```python
from build123d import *

# Parameters (mm, degrees)
SKETCH_1_R      = 1.65
EXTRUDE_1_DEPTH = 3


with BuildPart() as part:
    # 草图1 → 凸台-拉伸1 (new body)
    with BuildSketch(Plane.XY):
        Polygon((-55, 10), (-55, -10), (55, -10), (55, 10), (50, 50.05274288), (30, 50.05274288), (25.979309591, 25), (-25.864232627, 25), (-30, 50.05274288), (-50, 50.05274288), align=None)
        with Locations((15, 0)):
            Circle(SKETCH_1_R, mode=Mode.SUBTRACT)
        with Locations((-15, 0)):
            Circle(SKETCH_1_R, mode=Mode.SUBTRACT)
        with Locations((35, 0)):
            Circle(SKETCH_1_R, mode=Mode.SUBTRACT)
        with Locations((-35, 0)):
            Circle(SKETCH_1_R, mode=Mode.SUBTRACT)
        with Locations((45, 0)):
            Circle(SKETCH_1_R, mode=Mode.SUBTRACT)
        with Locations((-45, 0)):
            Circle(SKETCH_1_R, mode=Mode.SUBTRACT)
        with Locations((-40, 20)):
            Circle(SKETCH_1_R, mode=Mode.SUBTRACT)
        with Locations((-40, 30)):
            Circle(SKETCH_1_R, mode=Mode.SUBTRACT)
        with Locations((40, 20)):
            Circle(SKETCH_1_R, mode=Mode.SUBTRACT)
        with Locations((40, 30)):
            Circle(SKETCH_1_R, mode=Mode.SUBTRACT)
        with Locations((-40, 40)):
            Circle(SKETCH_1_R, mode=Mode.SUBTRACT)
        with Locations((40, 40)):
            Circle(SKETCH_1_R, mode=Mode.SUBTRACT)
    extrude(amount=EXTRUDE_1_DEPTH)


solid = part.part
```
Source: CAD feature listing. Evaluate the final solid. Frame: model axes, mm. A direction names the side the tool comes from. Round coordinates to 2 decimals unless told otherwise and drop trailing zeros. Loops run counter-clockwise (first coordinate to the right, second up) from the corner with the lowest first, then second, coordinate; pieces in that order, holes last.
(1) Section query C-C (z = 2.15). Give the number of separate pieces and of enclosed holes in the cut face, and give its area (3 significant figures).
From the geometry:
separate pieces: 1
enclosed holes: 12
area: 4,900 mm2
(2) Section query A-A (x = -35). Output: boundary loops of the cut face in (y, z).
From the geometry:
outline: (-10, 0) - (-1.65, 0) - (-1.65, 3) - (-10, 3) - close; (1.65, 0) - (50.05, 0) - (50.05, 3) - (1.65, 3) - close
(3) Material intervals for probe 1 along Y at (x, z) = (40, 2.3); probe 2 along Y at (x, z) = (-15, 2.15); probe 3 along X at (y, z) = (28.5, 1.05), sorted ascending.
From the geometry:
probe 1: y = -10 to 18.35, 21.65 to 28.35, 31.65 to 38.35, 41.65 to 50.05
probe 2: y = -10 to -1.65, 1.65 to 25
probe 3: x = -52.69 to -40.69, -39.31 to -26.44, 26.54 to 39.31, 40.69 to 52.69
(4) Contact query for a flat-ended pin moving along its axis: pin 1 Ø3 at (x, y) = (-40, 40) entering from -Z. Output: stop coordinate, or through.
From the geometry:
pin 1: passes through
(5) Pull-direction query (X, two-part tool) for faces 1 (the flat face through (52.535, 29.746, 1.479)), 2 (the cylindrical face through (38.35, 20.07, 1.48)), 3 (the flat face through (-52.465, 30.307, 1.479)); classes: +X half, -X half, draft (parallel to the pull), parting line (faces both ways), or undercut.
From the geometry:
face 1: +X half
face 2: undercut
face 3: -X half
(6) Access query for faces 4 (the flat face through (28.018, 37.702, 1.479)), 5 (the cylindrical face through (-36.65, 0.07, 1.48)). Directions: +Z, -Z, +X, -X, +Y, -Y. A direction counts if a zero-diameter tool reaches every point of the face in a straight line with its end or side. Return the directions, or none.
From the geometry:
face 4: +Z, -Z, +Y
face 5: +Z, -Z
(7) Section query B-B (y = 0). Output: boundary loops of the cut face in (x, z).
From the geometry:
outline: (-55, 0) - (-46.65, 0) - (-46.65, 3) - (-55, 3) - close; (-43.35, 0) - (-36.65, 0) - (-36.65, 3) - (-43.35, 3) - close; (-33.35, 0) - (-16.65, 0) - (-16.65, 3) - (-33.35, 3) - close; (-13.35, 0) - (13.35, 0) - (13.35, 3) - (-13.35, 3) - close; (16.65, 0) - (33.35, 0) - (33.35, 3) - (16.65, 3) - close; (36.65, 0) - (43.35, 0) - (43.35, 3) - (36.65, 3) - close; (46.65, 0) - (55, 0) - (55, 3) - (46.65, 3) - close
(8) Section query D-D (x = 40). Output: boundary loops of the cut face in (y, z), and give its area (3 significant figures).
From the geometry:
outline: (-10, 0) - (18.35, 0) - (18.35, 3) - (-10, 3) - close; (21.65, 0) - (28.35, 0) - (28.35, 3) - (21.65, 3) - close; (31.65, 0) - (38.35, 0) - (38.35, 3) - (31.65, 3) - close; (41.65, 0) - (50.05, 0) - (50.05, 3) - (41.65, 3) - close
area: 150 mm2
